from build123d import *

# Parameters (mm, degrees)
BOSS_EXTRUDE1_DEPTH      = 1.5
BOSS_EXTRUDE1_DEPTH_BACK = 1.5
CUT_EXTRUDE1_START       = -0.5
CUT_EXTRUDE1_DEPTH       = 1
SKETCH3_R                = 2.5
BOSS_EXTRUDE2_DEPTH      = 0.5
BOSS_EXTRUDE3_START      = 0.5
SKETCH4_R                = 2.5
BOSS_EXTRUDE3_DEPTH      = 0.5


# Read off the part's stored shape, not the designer's step: Cut-Extrude1
with BuildPart() as part:
    # Sketch1 → Boss-Extrude1 (new, two sides: drawn at the far end of the back side and taken through both)
    with BuildSketch(Plane(origin=(0, 0, 0), x_dir=(1, 0, 0), z_dir=(0, 1, 0)).offset(-BOSS_EXTRUDE1_DEPTH_BACK)):
        with BuildLine():
            ThreePointArc((-3, -2.5), (0, -5.5), (3, -2.5))
            Line((3, -2.5), (3, 2.5))
            Line((3, 2.5), (0, 2.5))
            ThreePointArc((0, 2.5), (-2.192459912, 0.415475947), (-3, -2.5))
        make_face()
    extrude(amount=BOSS_EXTRUDE1_DEPTH + BOSS_EXTRUDE1_DEPTH_BACK)

    # Cut-Extrude1 outline → Cut-Extrude1 (cut)
    with BuildSketch(Plane(origin=(0, 0, 0), x_dir=(1, 0, 0), z_dir=(0, 1, 0)).offset(CUT_EXTRUDE1_START)):
        with BuildLine():
            ThreePointArc((3, -2.5), (2.771638598, -1.351949703), (2.121320344, -0.378679656))
            Line((2.121320344, -0.378679656), (-0.474039748, 2.216680435))
            ThreePointArc((-0.474039748, 2.216680435), (-2.328753609, 0.175235948), (-3, -2.5))
            ThreePointArc((-3, -2.5), (0, -5.5), (3, -2.5))
        make_face()
    extrude(amount=CUT_EXTRUDE1_DEPTH, mode=Mode.SUBTRACT)

    # Sketch3 → Boss-Extrude2 (add)
    with BuildSketch(Plane(origin=(0, 1.5, 0), x_dir=(1, 0, 0), z_dir=(0, 1, 0))):
        with Locations(Location((0, -2.5, 0), (0, 0, 270))):
            Circle(SKETCH3_R)
    extrude(amount=BOSS_EXTRUDE2_DEPTH)

    # Sketch4 → Boss-Extrude3 (add)
    with BuildSketch(Plane.XZ.offset(1.5).offset(BOSS_EXTRUDE3_START)):
        with Locations(Location((0, 2.5, 0), (0, 0, 90))):
            Circle(SKETCH4_R)
    extrude(amount=-BOSS_EXTRUDE3_DEPTH)


solid = part.part
Geometry check sheet. Reference: the model listing, model coordinates, mm. A direction names the side the tool comes from. Coordinates: 2 decimals unless noted, no trailing zeros. Loops run counter-clockwise (first coordinate to the right, second up) from the corner with the lowest first, then second, coordinate; pieces in that order, holes last. Notation, with made-up numbers: (41.25, 54.25) - (85.25, 54.25) arc R36 ccw to (85.25, 92.25) - close; hole circle Ø4 at (60, 37.25). An arc over 180 degrees is marked (long way). Use one line per item in the form item = value. Start each with the question number.
Item 1: Section check A-A, the plane x = -1.3. Enter the section's corners in (y, z).
Item 2: Mould release check, pull along Y, two halves, no side actions. Record for faces 5 (the face through (1, -1.5, 0)), 6 (the face through (0, 0.5, 2)), 7 (the face through (2.78, -0.01, 1.37)), 8 (the face through (0.1, 1.7, 0)): +Y half, -Y half, draft (parallel to the pull), parting line (faces both ways), or undercut.
Item 3: Thickness scan on probe 1 along Y at (x, z) = (0.35, 5.25); probe 2 along Y at (x, z) = (-1.9, 2); probe 3 along Y at (x, z) = (2.4, -0.5). Record the ranges inside material, lowest first.
Item 4: Section check D-D, the plane y = -1.1. Enter the section's corners in (x, z), and give its area (3 significant figures).
Item 5: Tool access check on faces 1 (the face through (-0.1, -1.8, 0)), 2 (the face through (0, 2, 2)), 3 (the face through (1, 1.5, 0)), 4 (the face through (0.84, -0.01, -0.9)). Record the directions out of +Z, -Z, +X, -X, +Y, -Y that give a thin tool (end or side, any length) a straight path to the whole face; none if there is none.
Item 6: Section check C-C, the plane z = 0.75. Enter the section's corners in (x, y).
Item 7: Gauge pin test, flat end, axial feed: pin 1 (1.5 mm diameter, centred on x = -1, y = 1, fed in from +Z). Record the tip position at first contact, or that the pin passes through.
Item 8: Section check B-B, the plane y = 0.4. Enter the section's corners in (x, z), and give its area (3 significant figures).
Computed:
q1.outline = (-2, 0.36) - (-1.5, 0.36) - (-1.5, -1.55) - (-0.5, -1.55) - (-0.5, 5.2) - (-1.5, 5.2) - (-1.5, 4.64) - (-2, 4.64) - close; (0.5, -1.55) - (1.5, -1.55) - (1.5, 0.36) - (2, 0.36) - (2, 4.64) - (1.5, 4.64) - (1.5, 5.2) - (0.5, 5.2) - close
q2.face_5 = -Y half
q2.face_6 = undercut
q2.face_7 = undercut
q2.face_8 = draft
q3.probe_1 = -1.5 to -0.5, 0.5 to 1.5
q3.probe_2 = -2 to -0.5, 0.5 to 2
q3.probe_3 = -1.5 to 1.5
q4.outline = (-3, 2.5) arc R5.67 ccw to (0, -2.5) - (3, -2.5) - (3, 2.5) arc R3 ccw to start
q4.area = 39.8 mm2
q5.face_1 = -Y
q5.face_2 = +Z, -Z, +X, -X, +Y
q5.face_3 = +Y
q5.face_4 = +Z, -X
q6.outline = (-2.72, -1.5) - (-1.79, -1.5) - (-1.79, -2) - (1.79, -2) - (1.79, -1.5) - (3, -1.5) - (3, 1.5) - (1.79, 1.5) - (1.79, 2) - (-1.79, 2) - (-1.79, 1.5) - (-2.72, 1.5) - (-2.72, 0.5) - (2.44, 0.5) - (2.44, -0.5) - (-2.72, -0.5) - close
q7.pin_1 = 5.49
q8.outline = (-0.47, -2.22) arc R5.67 ccw to (0, -2.5) - (3, -2.5) - (3, 2.5) arc R3 cw to (2.12, 0.38) - close
q8.area = 7.15 mm2
